Autodesk Inventor part; units mm, degrees
ref_plane "Work Plane2" through (0, 7, 0) normal (0, -1, 0) x (1, 0, 0)
ref_plane "Work Plane3" through (0.398, 0.0199, 35) normal (-0.0995, 0.995, 0) x (0.995, 0.0995, 0)
ref_plane "YZ Plane" through (0, 0, 0) normal (1, 0, 0) x (0, 1, 0)
sketch "Sketch1" plane through (0, 0, 0) normal (0, 0, 1) x (1, 0, 0)
  line L0 (0, 0) -> (30, 0)
  line L1 (30, 0) -> (30, 3)
  line L2 (30, 3) -> (0, 0)
  dimension "d0" = 30
  dimension "d1" = 3
extrude "Extrusion1" add sketch "Sketch1" along normal blind 35
sketch "Sketch2" plane through (0, 0, 0) normal (0, -1, 0) x (1, 0, 0)
  circle A0 centre (26.2, 15) radius 0.6
  line L0 (0, 35) -> (30, 35)
  line L1 (30, 0) -> (30, 35)
  circle A1 centre (20.2, 15) radius 0.6
  circle A2 centre (14.2, 15) radius 0.6
  circle A3 centre (8.2, 15) radius 0.6
  circle A4 centre (2.2, 15) radius 0.6
  circle A5 centre (27.2, 10) radius 0.6
  circle A6 centre (21.2, 10) radius 0.6
  circle A7 centre (15.2, 10) radius 0.6
  circle A8 centre (9.2, 10) radius 0.6
  circle A9 centre (3.2, 10) radius 0.6
  circle A10 centre (28.2, 5) radius 0.6
  circle A11 centre (22.2, 5) radius 0.6
  circle A12 centre (16.2, 5) radius 0.6
  circle A13 centre (10.2, 5) radius 0.6
  circle A14 centre (4.2, 5) radius 0.6
  line L2 (0, 0) -> (30, 0)
  circle A15 centre (25.2, 20) radius 0.6
  circle A16 centre (19.2, 20) radius 0.6
  circle A17 centre (13.2, 20) radius 0.6
  circle A18 centre (7.2, 20) radius 0.6
  circle A19 centre (1.2, 20) radius 0.6
  circle A20 centre (24.2, 25) radius 0.6
  circle A21 centre (18.2, 25) radius 0.6
  circle A22 centre (12.2, 25) radius 0.6
  circle A23 centre (6.2, 25) radius 0.6
  circle A24 centre (23.2, 30) radius 0.6
  circle A25 centre (17.2, 30) radius 0.6
  circle A26 centre (11.2, 30) radius 0.6
  circle A27 centre (5.2, 30) radius 0.6
  dimension "d4" = 1.2
  dimension "d6" = 3.8
  dimension "d9" = 6
  dimension "d14" = 1.2
  dimension "d16" = 1
  dimension "d17" = 5
  dimension "d20" = 6
  dimension "d25" = 1.2
  dimension "d26" = 1
  dimension "d27" = 5
  dimension "d30" = 6
  dimension "d87" = 5
  dimension "d88" = 1.2
  dimension "d89" = 5
  dimension "d90" = 1
  dimension "d93" = 6
  dimension "d109" = 1.2
  dimension "d110" = 5
  dimension "d111" = 1
  dimension "d114" = 6
  dimension "d119" = 1.2
  dimension "d120" = 1
  dimension "d121" = 5
  dimension "d124" = 6
extrude "Extrusion2" cut sketch "Sketch2" against normal through all
sketch "Sketch4" plane through (0, 0, 35) normal (0, 0, 1) x (1, 0, 0)
  line L0 (30, 3) -> (0, 0)
  line L1 (0, 0) -> (0, 4)
  line L2 (30, 0) -> (30, 3)
  line L3 (30, 3) -> (30, 7)
  line L4 (30, 7) -> (0, 4)
  line L5 (0, 0) -> (30, 3)
  dimension "d41" = 4
  dimension "d42" = 4
extrude "Extrusion4" add sketch "Sketch4" against normal blind 35
sketch "Sketch5" plane through (30, 0, 35) normal (1, 0, 0) x (0, 0, -1)
  line L0 (0, 7) -> (0, 4)
  line L1 (35, 0) -> (0, 0)
  line L2 (0, 0) -> (0, 7)
  line L3 (0, 7) -> (35, 7)
  line L4 (35, 7) -> (35, 0)
extrude "Extrusion5" add sketch "Sketch5" along normal blind 2
sketch "Sketch7" plane through (0, 0, 35) normal (-1, 0, 0) x (0, 0, 1)
  line L0 (0, 7) -> (0, 4)
  line L1 (0, 4) -> (-35, 4)
  line L2 (-35, 4) -> (-35, 0)
  line L3 (-35, 0) -> (0, 0)
  line L4 (0, 0) -> (0, 4)
extrude "Extrusion6" add sketch "Sketch7" along normal blind 2
ref_plane "Work Plane2" through (0, 7, 0) normal (0, -1, 0) x (1, 0, 0)
sketch "Sketch6" plane through (0, 7, 0) normal (0, -1, 0) x (1, 0, 0)
  circle A0 centre (26.2, 15) radius 1
  line L0 (0, 0) -> (30, 0)
  line L1 (30, 35) -> (30, 0)
  line L2 (30, 35) -> (0, 35)
  circle A1 centre (20.2, 15) radius 1
  circle A2 centre (14.2, 15) radius 1
  circle A3 centre (8.2, 15) radius 1
  circle A4 centre (2.2, 15) radius 1
  circle A5 centre (27.2, 10) radius 1
  circle A6 centre (21.2, 10) radius 1
  circle A7 centre (15.2, 10) radius 1
  circle A8 centre (9.2, 10) radius 1
  circle A9 centre (3.2, 10) radius 1
  circle A10 centre (28.2, 5) radius 1
  circle A11 centre (22.2, 5) radius 1
  circle A12 centre (16.2, 5) radius 1
  circle A13 centre (10.2, 5) radius 1
  circle A14 centre (4.2, 5) radius 1
  circle A15 centre (25.2, 20) radius 1
  circle A16 centre (19.2, 20) radius 1
  circle A17 centre (13.2, 20) radius 1
  circle A18 centre (7.2, 20) radius 1
  circle A19 centre (1.2, 20) radius 1
  circle A20 centre (24.2, 25) radius 1
  circle A21 centre (18.2, 25) radius 1
  circle A22 centre (12.2, 25) radius 1
  circle A23 centre (6.2, 25) radius 1
  circle A24 centre (23.2, 30) radius 1
  circle A25 centre (17.2, 30) radius 1
  circle A26 centre (11.2, 30) radius 1
  circle A27 centre (5.2, 30) radius 1
  dimension "d49" = 2
  dimension "d52" = 3.8
  dimension "d60" = 6
  dimension "d65" = 2
  dimension "d66" = 5
  dimension "d67" = 1
  dimension "d70" = 6
  dimension "d75" = 2
  dimension "d76" = 5
  dimension "d77" = 1
  dimension "d80" = 6
  dimension "d98" = 5
  dimension "d99" = 2
  dimension "d100" = 5
  dimension "d101" = 1
  dimension "d104" = 6
  dimension "d129" = 2
  dimension "d130" = 5
  dimension "d131" = 1
  dimension "d134" = 6
  dimension "d139" = 2
  dimension "d140" = 5
  dimension "d141" = 1
  dimension "d144" = 6
ref_plane "Work Plane3" through (0.398, 0.0199, 35) normal (-0.0995, 0.995, 0) x (0.995, 0.0995, 0)
extrude "Extrusion7" cut sketch "Sketch6" along normal up to surface surface through (0.398, 0.0199, 35) normal (-0.0995, 0.995, 0)
properties part number "FiberJig"
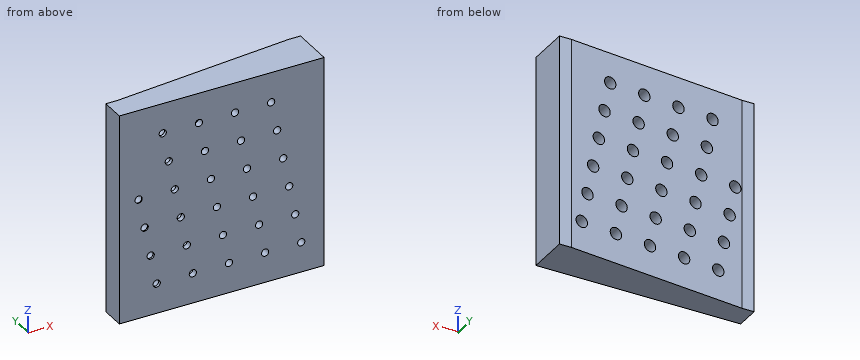
Read the model definition and answer for the solid it produces. Units are mm, in the model's axes. Coordinates: 2 decimals unless noted, no trailing zeros. Loops run counter-clockwise (first coordinate to the right, second up) from the corner with the lowest first, then second, coordinate; pieces in that order, holes last.
(1) Consider line 1 along X through (y, z) = (3.75, 20); line 2 along Z through (x, y) = (22.2, 1.6); line 3 along X through (y, z) = (1.75, 10). Determine where each line is inside the solid, lowest interval first.
Solution:
line 1: x = -2 to 0.2, 2.2 to 6.2, 8.2 to 12.2, 14.2 to 18.2, 20.2 to 24.2, 26.2 to 32
line 2: z = 0 to 4.4, 5.6 to 35
line 3: x = -2 to 2.2, 4.2 to 8.2, 10.2 to 14.2, 16.2 to 20.6, 21.8 to 26.6, 27.8 to 32
(2) The part is cut by section A-A (z = 13.5). Determine the outline of the cut face in (x, y), and give its area (3 significant figures).
Solution:
outline: (-2, 0) - (32, 0) - (32, 7) - (30, 7) - (0, 4) - (-2, 4) - close
area: 187 mm2
(3) The part is cut by section B-B (z = 30). Count the separate pieces of the cut face and the enclosed holes in it, and give its area (3 significant figures).
Solution:
separate pieces: 5
enclosed holes: 0
area: 148 mm2
(4) Flat-ended cylindrical pins translate along their axes: pin 1 Ø1.6 at (x, z) = (2.2, 15) entering from +Y; pin 2 Ø3 at (x, z) = (16.2, 5) entering from +Y; pin 3 Ø1 at (x, z) = (10.2, 5) entering from +Y; pin 4 Ø1.6 at (x, z) = (11.2, 30) entering from +Y. Find the tip coordinate at first contact, or state that the pin passes through.
Solution:
pin 1: stops at y = 0.28
pin 2: stops at y = 5.77
pin 3: passes through
pin 4: stops at y = 1.18
